```python
from build123d import *

# Parameters (mm, degrees)
ESQUISSE1_W             = 34
ESQUISSE1_H             = 86
BOSS_EXTRU_1_DEPTH      = 2
ESQUISSE2_W             = 30
ESQUISSE2_H             = 82
ESQUISSE2_W_2           = 26
ESQUISSE2_H_2           = 78
BOSS_EXTRU_2_DEPTH      = 4
CONG_3_R                = 1
CONG_2_R                = 2.5
ESQUISSE3_R             = 10
ENL_V_MAT_EXTRU_1_DEPTH = 4


with BuildPart() as part:
    # Esquisse1 → Boss.-Extru.1 (new body)
    with BuildSketch(Plane.XY):
        Rectangle(ESQUISSE1_W, ESQUISSE1_H)
    extrude(amount=BOSS_EXTRU_1_DEPTH)

    # Esquisse2 → Boss.-Extru.2 (add)
    with BuildSketch(Plane.XY.offset(2)):
        Rectangle(ESQUISSE2_W, ESQUISSE2_H)
        Rectangle(ESQUISSE2_W_2, ESQUISSE2_H_2, mode=Mode.SUBTRACT)
    extrude(amount=BOSS_EXTRU_2_DEPTH)

    # Congé3
    cong_3_edges = [part.edges().sort_by_distance(p)[0] for p in [
        (0, 43, 0),
        (17, 0, 0),
        (0, -43, 0),
        (-17, 0, 0),
    ]]
    fillet(cong_3_edges, radius=CONG_3_R)

    # Congé2
    # the kernel refuses this fillet: 2.5 mm, written as the material it adds along each edge
    with BuildSketch(Plane(origin=(-13, -39, 2), x_dir=(0, 1, 0), z_dir=(0, 0, 1)), Plane(origin=(13, 39, 2), x_dir=(0, -1, 0), z_dir=(0, 0, 1)), Plane(origin=(-13, 39, 2), x_dir=(1, 0, 0), z_dir=(0, 0, 1))) as cong_2_piece_1:
        with BuildLine():
            CenterArc((CONG_2_R, -CONG_2_R), CONG_2_R, 90, 90)
            Line((0, -CONG_2_R), (-CONG_2_R * 0.02, -CONG_2_R))
            Line((-CONG_2_R * 0.02, -CONG_2_R), (-CONG_2_R * 0.02, CONG_2_R * 0.02))
            Line((-CONG_2_R * 0.02, CONG_2_R * 0.02), (CONG_2_R, CONG_2_R * 0.02))
            Line((CONG_2_R, CONG_2_R * 0.02), (CONG_2_R, 0))
        make_face()
    extrude(amount=4)
    with BuildSketch(Plane(origin=(13, -39, 2), x_dir=(0, 1, 0), z_dir=(0, 0, 1))) as cong_2_piece_2:
        with BuildLine():
            CenterArc((CONG_2_R, CONG_2_R), CONG_2_R, 180, 90)
            Line((0, CONG_2_R), (-CONG_2_R * 0.02, CONG_2_R))
            Line((-CONG_2_R * 0.02, CONG_2_R), (-CONG_2_R * 0.02, -CONG_2_R * 0.02))
            Line((-CONG_2_R * 0.02, -CONG_2_R * 0.02), (CONG_2_R, -CONG_2_R * 0.02))
            Line((CONG_2_R, -CONG_2_R * 0.02), (CONG_2_R, 0))
        make_face()
    extrude(amount=4)
    # the kernel refuses this fillet: 2.5 mm, written as the material it takes off along each edge
    with BuildSketch(Plane(origin=(14.5, 40.5, 0), x_dir=(0, 1, 0), z_dir=(-1, 0, 0))) as cong_2_2_piece_1:
        with BuildLine():
            CenterArc((1.5, -1), 1, 0, 90)
            Line((2.5, -1), (2.5, 0))
            Line((2.5, 0), (1.5, 0))
        make_face()
    revolve(axis=Axis((14.5, 40.5, 0), (0, 0, -1)), revolution_arc=90, mode=Mode.SUBTRACT)
    with BuildSketch(Plane(origin=(14.5, -40.5, 0), x_dir=(1, 0, 0), z_dir=(0, 1, 0))) as cong_2_2_piece_2:
        with BuildLine():
            CenterArc((1.5, -1), 1, 0, 90)
            Line((2.5, -1), (2.5, 0))
            Line((2.5, 0), (1.5, 0))
        make_face()
    revolve(axis=Axis((14.5, -40.5, 0), (0, 0, -1)), revolution_arc=90, mode=Mode.SUBTRACT)
    with BuildSketch(Plane(origin=(-14.5, 40.5, 0), x_dir=(-1, 0, 0), z_dir=(0, -1, 0))) as cong_2_2_piece_3:
        with BuildLine():
            CenterArc((1.5, -1), 1, 0, 90)
            Line((2.5, -1), (2.5, 0))
            Line((2.5, 0), (1.5, 0))
        make_face()
    revolve(axis=Axis((-14.5, 40.5, 0), (0, 0, -1)), revolution_arc=90, mode=Mode.SUBTRACT)
    with BuildSketch(Plane(origin=(-14.5, -40.5, 0), x_dir=(0, -1, 0), z_dir=(1, 0, 0))) as cong_2_2_piece_4:
        with BuildLine():
            CenterArc((1.5, -1), 1, 0, 90)
            Line((2.5, -1), (2.5, 0))
            Line((2.5, 0), (1.5, 0))
        make_face()
    revolve(axis=Axis((-14.5, -40.5, 0), (0, 0, -1)), revolution_arc=90, mode=Mode.SUBTRACT)
    with BuildSketch(Plane(origin=(-15, 41, 2), x_dir=(0, -1, 0), z_dir=(0, 0, 1)), Plane(origin=(-15, -41, 2), x_dir=(1, 0, 0), z_dir=(0, 0, 1)), Plane(origin=(15, 41, 2), x_dir=(-1, 0, 0), z_dir=(0, 0, 1))) as cong_2_2_piece_5:
        with BuildLine():
            CenterArc((CONG_2_R, CONG_2_R), CONG_2_R, 180, 90)
            Line((0, CONG_2_R), (-CONG_2_R * 0.02, CONG_2_R))
            Line((-CONG_2_R * 0.02, CONG_2_R), (-CONG_2_R * 0.02, -CONG_2_R * 0.02))
            Line((-CONG_2_R * 0.02, -CONG_2_R * 0.02), (CONG_2_R, -CONG_2_R * 0.02))
            Line((CONG_2_R, -CONG_2_R * 0.02), (CONG_2_R, 0))
        make_face()
    extrude(amount=4, mode=Mode.SUBTRACT)
    with BuildSketch(Plane(origin=(15, -41, 2), x_dir=(-1, 0, 0), z_dir=(0, 0, 1))) as cong_2_2_piece_6:
        with BuildLine():
            CenterArc((CONG_2_R, -CONG_2_R), CONG_2_R, 90, 90)
            Line((0, -CONG_2_R), (-CONG_2_R * 0.02, -CONG_2_R))
            Line((-CONG_2_R * 0.02, -CONG_2_R), (-CONG_2_R * 0.02, CONG_2_R * 0.02))
            Line((-CONG_2_R * 0.02, CONG_2_R * 0.02), (CONG_2_R, CONG_2_R * 0.02))
            Line((CONG_2_R, CONG_2_R * 0.02), (CONG_2_R, 0))
        make_face()
    extrude(amount=4, mode=Mode.SUBTRACT)
    with BuildSketch(Plane(origin=(-17, 43, 0), x_dir=(0, -1, 0), z_dir=(0, 0, 1)), Plane(origin=(-17, -43, 0), x_dir=(1, 0, 0), z_dir=(0, 0, 1))) as cong_2_2_piece_7:
        with BuildLine():
            CenterArc((CONG_2_R, CONG_2_R), CONG_2_R, 180, 90)
            Line((0, CONG_2_R), (-CONG_2_R * 0.02, CONG_2_R))
            Line((-CONG_2_R * 0.02, CONG_2_R), (-CONG_2_R * 0.02, -CONG_2_R * 0.02))
            Line((-CONG_2_R * 0.02, -CONG_2_R * 0.02), (CONG_2_R, -CONG_2_R * 0.02))
            Line((CONG_2_R, -CONG_2_R * 0.02), (CONG_2_R, 0))
        make_face()
    extrude(amount=2, mode=Mode.SUBTRACT)
    with BuildSketch(Plane(origin=(17, 43, 0), x_dir=(0, -1, 0), z_dir=(0, 0, 1)), Plane(origin=(17, -43, 0), x_dir=(-1, 0, 0), z_dir=(0, 0, 1))) as cong_2_2_piece_8:
        with BuildLine():
            CenterArc((CONG_2_R, -CONG_2_R), CONG_2_R, 90, 90)
            Line((0, -CONG_2_R), (-CONG_2_R * 0.02, -CONG_2_R))
            Line((-CONG_2_R * 0.02, -CONG_2_R), (-CONG_2_R * 0.02, CONG_2_R * 0.02))
            Line((-CONG_2_R * 0.02, CONG_2_R * 0.02), (CONG_2_R, CONG_2_R * 0.02))
            Line((CONG_2_R, CONG_2_R * 0.02), (CONG_2_R, 0))
        make_face()
    extrude(amount=2, mode=Mode.SUBTRACT)

    # Esquisse3 → Enlèv. mat.-Extru.1 (cut)
    with BuildSketch(Plane(origin=(0, 0, 0), x_dir=(-1, 0, 0), z_dir=(0, 0, -1))):
        with Locations((0, -25.553422343)):
            Circle(ESQUISSE3_R)
    extrude(amount=-ENL_V_MAT_EXTRU_1_DEPTH, mode=Mode.SUBTRACT)


solid = part.part
```
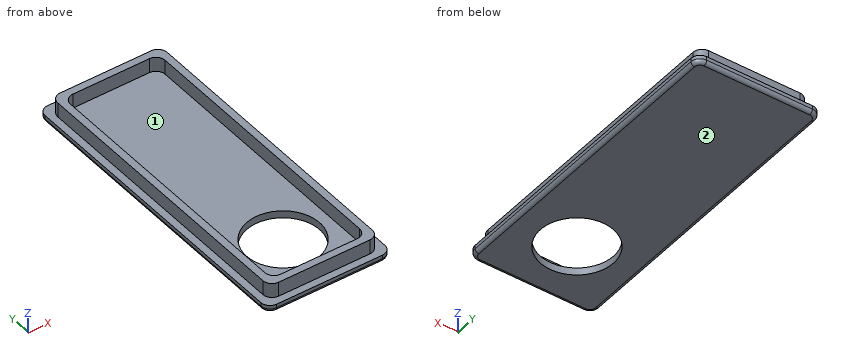
Work out the finished part from the listing and answer in its coordinate system (mm). Face numbers are marked on the shaded views. Round coordinates to 2 decimals unless told otherwise and drop trailing zeros. Loops run counter-clockwise (first coordinate to the right, second up) from the corner with the lowest first, then second, coordinate; pieces in that order, holes last.
(1) The part is cut by section D-D, the plane y = 15. Give the vertices of the cut face in (x, z), and give its area (3 significant figures).
Computed values:
outline: (-17, 1) arc R1 ccw to (-16, 0) - (16, 0) arc R1 ccw to (17, 1) - (17, 2) - (15, 2) - (15, 6) - (13, 6) - (13, 2) - (-13, 2) - (-13, 6) - (-15, 6) - (-15, 2) - (-17, 2) - close
area: 83.6 mm2
(2) The part is cut by section A-A, the plane x = 0. Give the vertices of the cut face in (y, z).
Computed values:
outline: (-43, 1) arc R1 ccw to (-42, 0) - (-35.55, 0) - (-35.55, 2) - (-39, 2) - (-39, 6) - (-41, 6) - (-41, 2) - (-43, 2) - close; (-15.55, 0) - (42, 0) arc R1 ccw to (43, 1) - (43, 2) - (41, 2) - (41, 6) - (39, 6) - (39, 2) - (-15.55, 2) - close
(3) The mould has two halves that part along Y. Classify the marked faces 1 and 2: pulls with the +Y half, pulls with the -Y half, needs draft (parallel to the pull), parting line crosses it, or undercut.
Computed values:
face 1: undercut
face 2: needs draft
(4) Each of these flat-tipped pins is pushed along its axis until it touches: P1, Ø1.2, axis at x = 2.5, z = 3.5, coming from the +Y side; P2, Ø1.5, axis at x = 11, z = 5, coming from the -Y side; P3, Ø2, axis at y = 11.5, z = 4.5, coming from the -X side. Where does it stop, or does it pass through?
Computed values:
P1: stops at y = 41
P2: stops at y = -41
P3: stops at x = -15
(5) The part is cut by section B-B, the plane z = 3.9. Give the vertices of the cut face in (x, y), and give its area (3 significant figures).
Computed values:
outline: (-15, -38.5) arc R2.5 ccw to (-12.5, -41) - (12.5, -41) arc R2.5 ccw to (15, -38.5) - (15, 38.5) arc R2.5 ccw to (12.5, 41) - (-12.5, 41) arc R2.5 ccw to (-15, 38.5) - close; hole (-13, -36.5) arc R2.5 ccw to (-10.5, -39) - (10.5, -39) arc R2.5 ccw to (13, -36.5) - (13, 36.5) arc R2.5 ccw to (10.5, 39) - (-10.5, 39) arc R2.5 ccw to (-13, 36.5) - close
area: 432 mm2
(6) Find the intervals of material crossed by L1, parallel to Y at x = 0, z = 0.85; L2, parallel to Y at x = 7.5, z = 4.4; L3, parallel to X at y = 23, z = 2.5, in increasing order.
Computed values:
L1: y = -42.99 to -35.55, -15.55 to 42.99
L2: y = -41 to -39, 39 to 41
L3: x = -15 to -13, 13 to 15
(7) The part is cut by section C-C, the plane y = -21.5. Give the vertices of the cut face in (x, z), and give its area (3 significant figures).
Computed values:
outline: (-17, 1) arc R1 ccw to (-16, 0) - (-9.14, 0) - (-9.14, 2) - (-13, 2) - (-13, 6) - (-15, 6) - (-15, 2) - (-17, 2) - close; (9.14, 0) - (16, 0) arc R1 ccw to (17, 1) - (17, 2) - (15, 2) - (15, 6) - (13, 6) - (13, 2) - (9.14, 2) - close
area: 47.0 mm2
